Part model, mm, in its own coordinate system. Round coordinates to 2 decimals unless told otherwise and drop trailing zeros. Write each loop counter-clockwise with the first axis right and the second up, starting at its lowest first coordinate (ties: lowest second). Pieces come first, ordered by that corner, then holes. Notation, with made-up numbers: (69.25, 74) -> (95.25, 74) arc R27 cw to (95.25, 112) -> close; hole circle Ø11 at (25.5, 53.5). An arc over 180 degrees is marked (long way). Return JSON: item names as keys, results as strings. Group by question number.
```python
from build123d import *

# Parameters (mm, degrees)
SALIENTE_EXTRUIR1_DEPTH = 6.35
CROQUIS3_W              = 446.786
CROQUIS3_H              = 39.37
CORTAR_EXTRUIR1_DEPTH   = 246.599940908
REDONDEO2_R             = 2.54


with BuildPart() as part:
    # Croquis2 → Saliente-Extruir1 (new body)
    with BuildSketch(Plane.XY):
        Polygon((-242.443, -38.735), (-242.443, 38.735), (223.393, 38.735), (223.393, 19.685), (223.393, -19.685), (223.393, -38.735), align=None)
    extrude(amount=SALIENTE_EXTRUIR1_DEPTH)

    # Croquis3 → Cortar-Extruir1 (cut, through all)
    with BuildSketch(Plane.XY.offset(6.35)):
        Rectangle(CROQUIS3_W, CROQUIS3_H)
    extrude(amount=-CORTAR_EXTRUIR1_DEPTH, mode=Mode.SUBTRACT)

    # Redondeo2
    redondeo2_edges = [part.edges().sort_by_distance(p)[0] for p in [
        (223.393, -38.735, 3.175),
        (-242.443, -38.735, 3.175),
        (-242.443, 38.735, 3.175),
        (223.393, 38.735, 3.175),
        (223.393, 19.685, 3.175),
        (223.393, -19.685, 3.175),
    ]]
    fillet(redondeo2_edges, radius=REDONDEO2_R)


solid = part.part
```
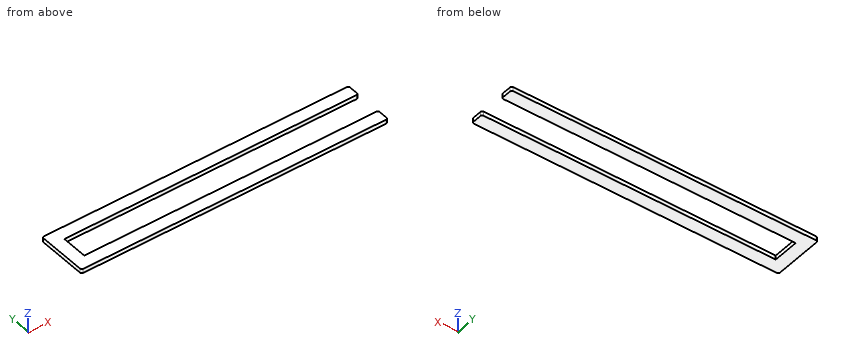
Item 1: Cut at A-A (x = -72). Write the cut outline in (y, z) (3 decimals), then the cut area to 3 significant figures.
Item 2: Cut at C-C (y = 14). Write the cut outline in (x, z), then the cut area to 3 significant figures.
Item 3: Cut at B-B (z = 2.75). Write the cut outline in (x, y) (3 decimals).
Item 4: Wall check: L1, parallel to Y at x = 10, z = 4.5 (3 decimals); L2, parallel to X at y = 1, z = 1.5. Give the ranges that are in metal, low to high.
Checks:
{
 "1": {"outline": "(-38.735, 0) -> (-19.685, 0) -> (-19.685, 6.35) -> (-38.735, 6.35) -> close; (19.685, 0) -> (38.735, 0) -> (38.735, 6.35) -> (19.685, 6.35) -> close", "area": "242 mm2"},
 "2": {"outline": "(-242.44, 0) -> (-223.39, 0) -> (-223.39, 6.35) -> (-242.44, 6.35) -> close", "area": "121 mm2"},
 "3": {"outline": "(-242.443, -36.195) arc R2.54 ccw to (-239.903, -38.735) -> (220.853, -38.735) arc R2.54 ccw to (223.393, -36.195) -> (223.393, -22.225) arc R2.54 ccw to (220.853, -19.685) -> (-223.393, -19.685) -> (-223.393, 19.685) -> (220.853, 19.685) arc R2.54 ccw to (223.393, 22.225) -> (223.393, 36.195) arc R2.54 ccw to (220.853, 38.735) -> (-239.903, 38.735) arc R2.54 ccw to (-242.443, 36.195) -> close"},
 "4": {"L1": "y = -38.735 to -19.685, 19.685 to 38.735", "L2": "x = -242.44 to -223.39"}
}
